Could you check a few things on this model? Use its own coordinates, in mm. Face numbers are marked on the shaded views. Coordinates: 2 decimals unless noted, no trailing zeros. Loops run counter-clockwise (first coordinate to the right, second up) from the corner with the lowest first, then second, coordinate; pieces in that order, holes last.
from build123d import *

# Parameters (mm, degrees)
SKETCH1_R           = 42.8625
SKETCH1_R_2         = 11.1125
BOSS_EXTRUDE1_DEPTH = 9.525
SKETCH2_R           = 7.9375
CUT_EXTRUDE1_DEPTH  = 7.62
SKETCH3_W           = 3.683
SKETCH3_H           = 25.4
CUT_EXTRUDE2_DEPTH  = 3.429


with BuildPart() as part:
    # Sketch1 → Boss-Extrude1 (new body, symmetric)
    with BuildSketch(Plane.XY):
        Circle(SKETCH1_R)
        with Locations((0, 24.13)):
            Circle(SKETCH1_R_2, mode=Mode.SUBTRACT)
        with Locations((-20.897192993, -12.065)):
            Circle(SKETCH1_R_2, mode=Mode.SUBTRACT)
        with Locations((20.897192993, -12.065)):
            Circle(SKETCH1_R_2, mode=Mode.SUBTRACT)
    extrude(amount=BOSS_EXTRUDE1_DEPTH, both=True)

    # Sketch2 → Cut-Extrude1 (cut)
    with BuildSketch(Plane.XY.offset(9.525)):
        Circle(SKETCH2_R)
    extrude(amount=-CUT_EXTRUDE1_DEPTH, mode=Mode.SUBTRACT)

    # Sketch3 → Cut-Extrude2 (cut)
    with BuildSketch(Plane.XY.offset(9.525)):
        with Locations((0, -1.27)):
            Rectangle(SKETCH3_W, SKETCH3_H)
    extrude(amount=-CUT_EXTRUDE2_DEPTH, mode=Mode.SUBTRACT)


solid = part.part
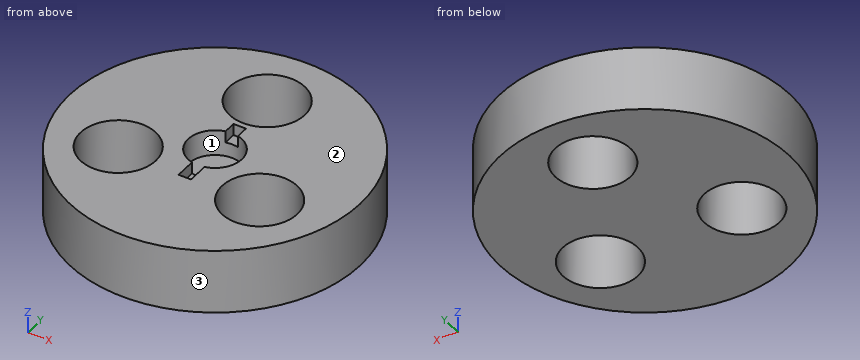
1) We'd pull the mould along X, two halves only. Please class the marked faces 1, 2 and 3: released by +X, released by -X, zero draft, split by the parting line, or undercut.
2) Imagine slicing it at A-A on x = 0. List the corners of the cut face in (y, z) for me (1 decimal), plus the area to 3 significant figures.
3) Imagine slicing it at D-D on z = -4.75. List the corners of the cut face in (x, y) for me (1 decimal), plus the area to 3 significant figures.
4) Will these pins go through, and if not, where does the flat tip stop? pin 1 (2.5 mm diameter, centred on y = 10.5, z = 8.5, fed in from +X); pin 2 (1.5 mm diameter, centred on y = 28.5, z = 5, fed in from +X); pin 3 (5 mm diameter, centred on x = 3.5, y = 0.5, fed in from +Z) (3 decimals); pin 4 (12 mm diameter, centred on x = 14.5, y = -12, fed in from -Z) (3 decimals).
5) Imagine slicing it at B-B on y = 24.13. List the corners of the cut face in (x, z) for me (1 decimal).
6) If I drill on L1, parallel to X at y = -19, z = 3.75; L2, parallel to Y at x = 0, z = 5.75; L3, parallel to X at y = -10.5, z = 3.75, over which ranges is the centre line in solid material (lowest first)?
7) Imagine slicing it at C-C on y = -5. List the corners of the cut face in (x, z) for me (3 decimals), plus the area to 3 significant figures.
Solved:
1. face 1: undercut
1. face 2: zero draft
1. face 3: split by the parting line
2. outline: (-42.9, -9.5) - (13, -9.5) - (13, 9.5) - (11.4, 9.5) - (11.4, 6.1) - (7.9, 6.1) - (7.9, 1.9) - (-7.9, 1.9) - (-7.9, 6.1) - (-14, 6.1) - (-14, 9.5) - (-42.9, 9.5) - close; (35.2, -9.5) - (42.9, -9.5) - (42.9, 9.5) - (35.2, 9.5) - close
2. area: 1,060 mm2
3. outline: circle Ø85.7 at (0, 0); hole circle Ø22.2 at (-20.9, -12.1); hole circle Ø22.2 at (0, 24.1); hole circle Ø22.2 at (20.9, -12.1)
3. area: 4,610 mm2
4. pin 1: stops at x = 41.85
4. pin 2: stops at x = 32.67
4. pin 3: stops at z = 1.905
4. pin 4: stops at z = -9.525
5. outline: (-35.4, -9.5) - (-11.1, -9.5) - (-11.1, 9.5) - (-35.4, 9.5) - close; (11.1, -9.5) - (35.4, -9.5) - (35.4, 9.5) - (11.1, 9.5) - close
6. L1: x = -38.42 to -29.58, -12.21 to 12.21, 29.58 to 38.42
6. L2: y = -42.86 to -7.94, 7.94 to 13.02, 35.24 to 42.86
6. L3: x = -41.56 to -31.9, -9.9 to 9.9, 31.9 to 41.56
7. outline: (-42.57, -9.525) - (-29.475, -9.525) - (-29.475, 9.525) - (-42.57, 9.525) - close; (-12.32, -9.525) - (12.32, -9.525) - (12.32, 9.525) - (6.165, 9.525) - (6.165, 1.905) - (-6.165, 1.905) - (-6.165, 9.525) - (-12.32, 9.525) - close; (29.475, -9.525) - (42.57, -9.525) - (42.57, 9.525) - (29.475, 9.525) - close
7. area: 874 mm2
